The model under review builds one solid part; all positions refer to its coordinate system, in mm. Face numbers are marked on the shaded views. A direction names the side the tool comes from. Round coordinates to 2 decimals unless told otherwise and drop trailing zeros. Loops run counter-clockwise (first coordinate to the right, second up) from the corner with the lowest first, then second, coordinate; pieces in that order, holes last. Notation, with made-up numbers: M 23.5,61.25 L 71.5,61.25 A34 cw 71.5,99.25 Z; hole C -23.75,64 d8. An arc over 180 degrees is marked long. Return JSON: item names as keys, results as strings. Group by question number.
Q1. Draft analysis for pull direction Y (two halves, no side actions). For the marked faces 4, 5 and 6, state which applies: pulls with the +Y half, pulls with the -Y half, needs draft (parallel to the pull), parting line crosses it, or undercut.
Q2. Clearance check with flat-ended pins moving along their axes: pin 1 Ø1.5 at (x, y) = (19, -76) entering from -Z; pin 2 Ø4 at (x, y) = (22, -119.5) entering from -Z; pin 3 Ø1 at (y, z) = (-92.5, 48) entering from -X. State where each tip first meets the part, or that it passes through.
Q3. Consider section B-B (y = -19.05). State the section outline as (x, z) points (3 decimals).
Q4. For the marked faces 1, 2 and 3, list the 3-axis set-ups (+Z, -Z, +X, -X, +Y, -Y) from which the entire face can be reached by the end or side of a thin tool; tool diameter is ignored.
Q5. Consider section C-C (z = -13.5). State the section outline as (x, y) points.
Q6. To check wall thickness, follow line 1 along Y through (x, z) = (37.5, 41); line 2 along Z through (x, y) = (42.75, -19.05) (3 decimals); line 3 along Y through (x, z) = (39, -6). State the ranges of each line that lie inside material, in increasing order.
Q7. Consider section A-A (x = 38.1). Count the separate pieces of the cut face and the enclosed holes in it, and give its area (3 significant figures).
Q8. Consider section D-D (y = -91). State the section outline as (x, z) points, and give its area (3 significant figures).
from build123d import *

# Parameters (mm, degrees)
F1_DEPTH       = 139.7
F2_DEPTH       = 63.5
F3_R           = 25.4
F5_D           = 19.05
F5_CBORE_D     = 31.75
F5_CBORE_DEPTH = 25.4
F7_D           = 12.7


with BuildPart() as f1:
    # F0 (on Front) → F1 (new body)
    with BuildSketch(Plane.XZ):
        with BuildLine():
            Line((0, 44.45), (0, 0))
            Line((0, 0), (50.8, 31.75))
            Line((50.8, 31.75), (50.8, 69.85))
            Line((50.8, 69.85), (25.4, 69.85))
            ThreePointArc((25.4, 69.85), (7.439488, 62.410512), (0, 44.45))
        make_face()
    extrude(amount=F1_DEPTH)

    # F0 (on Front) → F2 (join)
    with BuildSketch(Plane.XZ):
        Polygon((50.8, 31.75), (0, 0), (0, -31.75), (50.8, -31.75), align=None)
    extrude(amount=F2_DEPTH)

    # F3
    f3_edges = [f1.edges().sort_by_distance(p)[0] for p in [
        (25.4, -63.5, -31.75),
    ]]
    fillet(f3_edges, radius=F3_R)

    # F5 (through all)
    with Locations(Plane.YZ.offset(50.8)):
        with Locations((-19.05, -6.35)):
            CounterBoreHole(F5_D / 2, F5_CBORE_D / 2, F5_CBORE_DEPTH)

    # F7 (through all)
    with Locations(Plane.XY.offset(69.85)):
        with Locations((38.1, -114.3)):
            Hole(F7_D / 2)


solid = f1.part
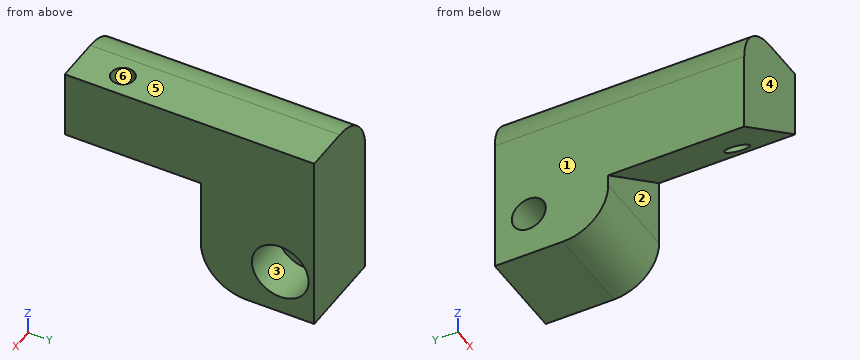
Values:
{
 "1": {"face 4": "pulls with the -Y half", "face 5": "needs draft", "face 6": "undercut"},
 "2": {"pin 1": "stops at z = 11.41", "pin 2": "stops at z = 12.5", "pin 3": "stops at x = 0.18"},
 "3": {"outline": "M 0,-31.75 L 50.8,-31.75 L 50.8,-22.225 L 25.4,-22.225 L 25.4,-15.875 L 0,-15.875 Z; M 0,3.175 L 25.4,3.175 L 25.4,9.525 L 50.8,9.525 L 50.8,69.85 L 25.4,69.85 A25.4 ccw 0,44.45 Z"},
 "4": {"face 1": "+Z, -Z, -X, +Y, -Y", "face 2": "-Z, +X, -Y", "face 3": "+X"},
 "5": {"outline": "M 0,-62.47 L 50.8,-62.47 L 50.8,-33.22 L 25.4,-33.22 L 25.4,-25.34 L 0,-25.34 Z; M 0,-12.76 L 25.4,-12.76 L 25.4,-4.88 L 50.8,-4.88 L 50.8,0 L 0,0 Z"},
 "6": {"line 1": "y = -139.7 to -120.62, -107.98 to 0", "line 2": "z = -31.75 to -22.225, 9.525 to 69.85", "line 3": "y = -63.5 to -34.92, -3.18 to 0"},
 "7": {"separate pieces": "2", "enclosed holes": "1", "area": "8,440 mm2"},
 "8": {"outline": "M 0,0 L 50.8,31.75 L 50.8,69.85 L 25.4,69.85 A25.4 ccw 0,44.45 Z", "area": "2,600 mm2"}
}
